Check sheet for the modelled part. Datum: model origin and axes. Units: mm. A direction names the side the tool comes from. Coordinates: 2 decimals unless noted, no trailing zeros. Loops run counter-clockwise (first coordinate to the right, second up) from the corner with the lowest first, then second, coordinate; pieces in that order, holes last.
```python
from build123d import *

# Parameters (mm, degrees)
CROQUIS1_W              = 30
CROQUIS1_H              = 30
SALIENTE_EXTRUIR1_DEPTH = 30
CROQUIS2_W              = 26
CROQUIS2_H              = 30
CORTAR_EXTRUIR1_DEPTH   = 26
CROQUIS3_R              = 1.55
CORTAR_EXTRUIR2_DEPTH   = 4
CROQUIS4_R              = 1.55
CORTAR_EXTRUIR3_DEPTH   = 4
CORTAR_EXTRUIR5_DEPTH   = 1
SALIENTE_EXTRUIR2_DEPTH = 2.5
SALIENTE_EXTRUIR3_DEPTH = 2.5
CROQUIS9_R              = 2.8
CORTAR_EXTRUIR6_DEPTH   = 1.5
REDONDEO1_R             = 5
REDONDEO2_R             = 3
REDONDEO3_R             = 2


with BuildPart() as part:
    # Croquis1 → Saliente-Extruir1 (new body)
    with BuildSketch(Plane(origin=(0, 0, 0), x_dir=(1, 0, 0), z_dir=(0, 1, 0))):
        with Locations((15, 15)):
            Rectangle(CROQUIS1_W, CROQUIS1_H)
    extrude(amount=SALIENTE_EXTRUIR1_DEPTH)

    # Croquis2 → Cortar-Extruir1 (cut)
    with BuildSketch(Plane(origin=(0, 30, 0), x_dir=(1, 0, 0), z_dir=(0, 1, 0))):
        with Locations((17, 15)):
            Rectangle(CROQUIS2_W, CROQUIS2_H)
    extrude(amount=-CORTAR_EXTRUIR1_DEPTH, mode=Mode.SUBTRACT)

    # Croquis3 → Cortar-Extruir2 (cut)
    with BuildSketch(Plane(origin=(4, 0, 0), x_dir=(0, 0, -1), z_dir=(1, 0, 0))):
        with Locations((15, 15)):
            Circle(CROQUIS3_R)
    extrude(amount=-CORTAR_EXTRUIR2_DEPTH, mode=Mode.SUBTRACT)

    # Croquis4 → Cortar-Extruir3 (cut)
    with BuildSketch(Plane(origin=(0, 4, 0), x_dir=(1, 0, 0), z_dir=(0, 1, 0))):
        with Locations((15, 15)):
            Circle(CROQUIS4_R)
    extrude(amount=-CORTAR_EXTRUIR3_DEPTH, mode=Mode.SUBTRACT)

    # Croquis6 → Cortar-Extruir5 (cut)
    with BuildSketch(Plane(origin=(4, 0, 0), x_dir=(0, 0, -1), z_dir=(1, 0, 0))):
        Polygon((11.651368439, 15), (13.325684219, 12.1), (16.674315781, 12.1), (18.348631561, 15), (16.674315781, 17.9), (13.325684219, 17.9), align=None)
    extrude(amount=-CORTAR_EXTRUIR5_DEPTH, mode=Mode.SUBTRACT)

    # Croquis7 → Saliente-Extruir2 (add)
    with BuildSketch(Plane.XY):
        with BuildLine():
            Line((25, 4), (4, 4))
            Line((4, 4), (4, 25))
            ThreePointArc((4, 25), (11.719105156, 11.719105156), (25, 4))
        make_face()
    extrude(amount=-SALIENTE_EXTRUIR2_DEPTH)

    # Croquis8 → Saliente-Extruir3 (add)
    with BuildSketch(Plane(origin=(0, 0, -30), x_dir=(-1, 0, 0), z_dir=(0, 0, -1))):
        with BuildLine():
            Line((-25, 4), (-4, 4))
            Line((-4, 4), (-4, 25))
            ThreePointArc((-4, 25), (-11.719105156, 11.719105156), (-25, 4))
        make_face()
    extrude(amount=-SALIENTE_EXTRUIR3_DEPTH)

    # Croquis9 → Cortar-Extruir6 (cut)
    with BuildSketch(Plane(origin=(0, 4, 0), x_dir=(1, 0, 0), z_dir=(0, 1, 0))):
        with Locations((15, 15)):
            Circle(CROQUIS9_R)
    extrude(amount=-CORTAR_EXTRUIR6_DEPTH, mode=Mode.SUBTRACT)

    # Redondeo1
    redondeo1_edges = [part.edges().sort_by_distance(p)[0] for p in [
        (4, 4, -15),
    ]]
    fillet(redondeo1_edges, radius=REDONDEO1_R)

    # Redondeo2
    redondeo2_edges = [part.edges().sort_by_distance(p)[0] for p in [
        (2, 30, -30),
        (30, 2, -30),
        (30, 2, 0),
        (30, 4, -15),
        (4, 30, -15),
        (2, 30, 0),
    ]]
    fillet(redondeo2_edges, radius=REDONDEO2_R)

    # Redondeo3
    redondeo3_edges = [part.edges().sort_by_distance(p)[0] for p in [
        (4, 17, -2.5),
        (17, 4, -27.5),
        (17, 4, -2.5),
        (5.464466094, 5.464466094, -2.5),
        (4, 17, -27.5),
        (5.464466094, 5.464466094, -27.5),
    ]]
    fillet(redondeo3_edges, radius=REDONDEO3_R)


solid = part.part
```
1) Set-up check for faces 5 (the flat face through (10, 10, -2.5)), 6 (the flat face through (3.507, 13.57, -12.477)), 7 (the flat face through (16.21, 2.5, -13.79)): record each of +Z, -Z, +X, -X, +Y, -Y from which the full face is reachable in a straight line by a thin tool's end or side.
Answer sheet:
face 5: +X, +Y
face 6: +X
face 7: +Y
2) Section check B-B on x = 15. Enter the section's corners in (y, z).
Answer sheet:
outline: (0, -30) - (8.88, -30) - (8.88, -27.5) - (6, -27.5) arc R2 cw to (4, -25.5) - (4, -17.8) - (2.5, -17.8) - (2.5, -16.55) - (0, -16.55) - close; (0, -13.45) - (2.5, -13.45) - (2.5, -12.2) - (4, -12.2) - (4, -4.5) arc R2 cw to (6, -2.5) - (8.88, -2.5) - (8.88, 0) - (0, 0) - close
3) Depth check by flat-ended pin: pin 1 (4 mm diameter, centred on x = 7, z = -25.5, fed in from -Y); pin 2 (0.8 mm diameter, centred on x = 3.5, z = -15.5, fed in from +Y); pin 3 (6 mm diameter, centred on x = 16, z = -14, fed in from +Y); pin 4 (9 mm diameter, centred on x = 21, z = -21.5, fed in from +Y). Enter the tip coordinate at first touch or a pass-through.
Answer sheet:
pin 1: stops at y = 0
pin 2: stops at y = 29.14
pin 3: stops at y = 4
pin 4: stops at y = 4.06
4) Section check A-A on z = -15. Enter the section's corners in (x, y).
Answer sheet:
outline: (0, 0) - (13.45, 0) - (13.45, 2.5) - (12.2, 2.5) - (12.2, 4) - (9, 4) arc R5 cw to (4, 9) - (4, 12.1) - (3, 12.1) - (3, 13.45) - (0, 13.45) - close; (0, 16.55) - (3, 16.55) - (3, 17.9) - (4, 17.9) - (4, 27) arc R3 ccw to (1, 30) - (0, 30) - close; (16.55, 0) - (30, 0) - (30, 1) arc R3 ccw to (27, 4) - (17.8, 4) - (17.8, 2.5) - (16.55, 2.5) - close
5) Section check D-D on x = 2. Enter the section's corners in (y, z).
Answer sheet:
outline: (0, -30) - (27, -30) arc R3 ccw to (29.83, -28) - (29.83, -2) arc R3 ccw to (27, 0) - (0, 0) - close; hole circle Ø3.1 at (15, -15)
6) Scan lines: line 1 (Z direction, x = 15, y = 1.35); line 2 (Z direction, x = 15, y = 3.65); line 3 (Y direction, x = 26.75, z = -26). Record each from-to range of solid material in increasing order.
Answer sheet:
line 1: z = -30 to -16.55, -13.45 to 0
line 2: z = -30 to -17.8, -12.2 to 0
line 3: y = 0 to 4
7) Mould release check, pull along Z, two halves, no side actions. Record for faces 1 (the flat face through (0, 15, -11)), 2 (the flat face through (10, 10, -27.5)), 3 (the flat face through (3.5, 17.9, -15)), 4 (the cylindrical face through (28.69, 1.58, -0.52)): +Z half, -Z half, draft (parallel to the pull), parting line (faces both ways), or undercut.
Answer sheet:
face 1: draft
face 2: undercut
face 3: undercut
face 4: +Z half
8) Section check C-C on z = -25. Enter the section's corners in (x, y), plus the area to 3 significant figures.
Answer sheet:
outline: (0, 0) - (30, 0) - (30, 1) arc R3 ccw to (27, 4) - (9, 4) arc R5 cw to (4, 9) - (4, 27) arc R3 ccw to (1, 30) - (0, 30) - close
area: 226 mm2
